Part print with two shaded views. Sizes in mm from the minimum x, y, z corner. A direction names the side the tool comes from. Round coordinates to 2 decimals unless told otherwise and drop trailing zeros. Order: outer loops, then holes, each group sorted by start corner. A loop starts at its lowest first (then second) coordinate and runs counter-clockwise, first axis right, second up. Notation, with made-up numbers: (14.5, -21.5) -> (23.5, -21.5) arc R27 cw to (23.5, -5.5) -> close; hole circle Ø3 at (6, 29). An arc over 180 degrees is marked (long way). Answer as a JSON object with one key per item and string values.
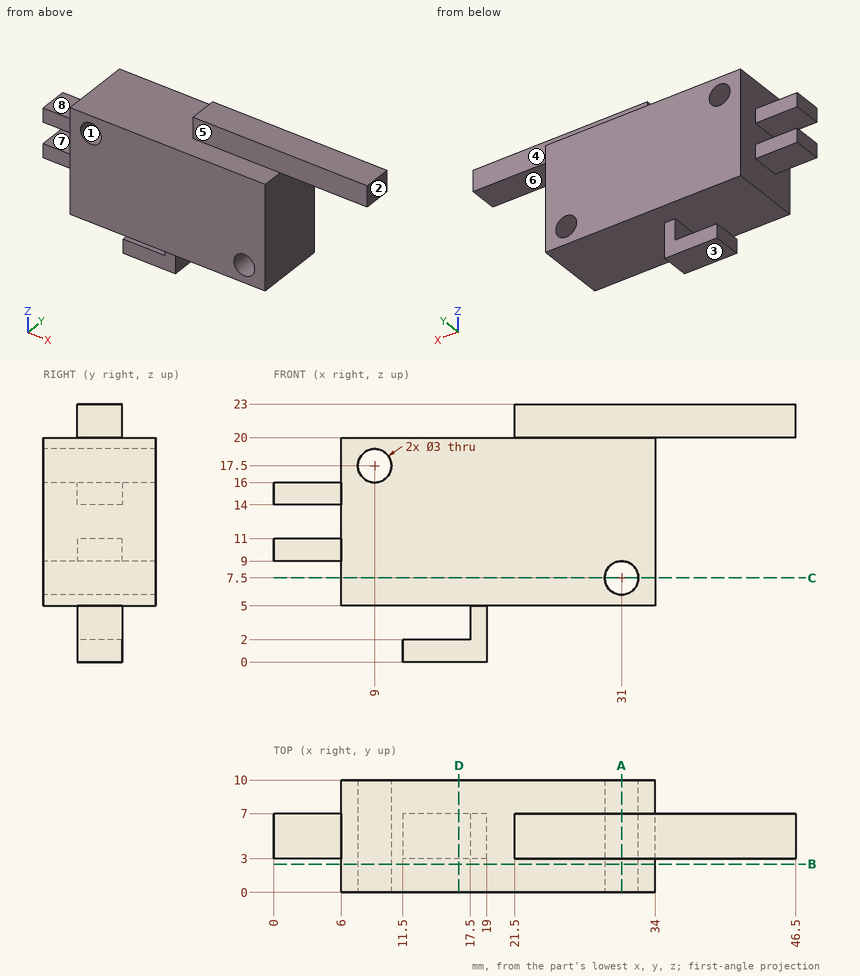
1) Cut at D-D, the plane x = 16.5. Give the cut face in (y, z).
Checked values:
{"outline": "(0, 5) -> (10, 5) -> (10, 20) -> (0, 20) -> close; (3, 0) -> (7, 0) -> (7, 2) -> (3, 2) -> close"}
2) Probe L1, parallel to Z at x = 31, y = 6.25; L2, parallel to Z at x = 9, y = 7.25; L3, parallel to X at y = 6, z = 17.5. List the from-to ranges inside material, lowest first. Write a range as from..to.
Checked values:
{"L1": "z = 5..6, 9..23", "L2": "z = 5..16, 19..20", "L3": "x = 6..7.5, 10.5..34"}
3) Cut at B-B, the plane y = 2.5. Give the cut face in (x, z).
Checked values:
{"outline": "(6, 5) -> (34, 5) -> (34, 20) -> (6, 20) -> close; hole circle Ø3 at (9, 17.5); hole circle Ø3 at (31, 7.5)"}
4) Cut at A-A, the plane x = 31. Give the cut face in (y, z), plus the area to 3 significant figures.
Checked values:
{"outline": "(0, 5) -> (10, 5) -> (10, 6) -> (0, 6) -> close; (0, 9) -> (10, 9) -> (10, 20) -> (7, 20) -> (7, 23) -> (3, 23) -> (3, 20) -> (0, 20) -> close", "area": "132 mm²"}
5) Flat gauge pins, fed straight in: pin 1 Ø2 at (y, z) = (8.5, 15.5) entering from -X; pin 2 Ø1.2 at (y, z) = (5, 3.5) entering from +X; pin 3 Ø2.5 at (x, z) = (33.5, 22) entering from -Y; pin 4 Ø2.5 at (x, z) = (31, 7.5) entering from +Y. Where does each tip first touch, or does it go through?
Checked values:
{"pin 1": "stops at x = 6", "pin 2": "stops at x = 19", "pin 3": "stops at y = 3", "pin 4": "passes through"}
6) Cut at C-C, the plane z = 7.5. Give the cut face in (x, y).
Checked values:
{"outline": "(6, 0) -> (29.5, 0) -> (29.5, 10) -> (6, 10) -> close; (32.5, 0) -> (34, 0) -> (34, 10) -> (32.5, 10) -> close"}
7) Which spindle directions (+Z, -Z, +X, -X, +Y, -Y) get a long thin tool onto all of the face, cutting with end or side? Do the marked faces 4, 5, 6, 7 and 8. Say none if no direction does.
Checked values:
{"face 4": "+Z, +X, -X, +Y", "face 5": "+Z, +X, -X, -Y", "face 6": "-Z, +X, +Y, -Y", "face 7": "-X, +Y, -Y", "face 8": "+Z, -X, +Y, -Y"}
8) Pull direction X, two halves, no side cores. Call the marked faces 1, 2 and 3: pulls with the +X half, pulls with the -X half, needs draft (parallel to the pull), parting line crosses it, or undercut.
Checked values:
{"face 1": "undercut", "face 2": "pulls with the +X half", "face 3": "needs draft"}
